from build123d import *

# Parameters (mm, degrees)
F0_R        = 3.81
F1_DEPTH    = 3.175
F2_R        = 10.16
F3_R        = 6.35
F4_T1_DEPTH = 25.1335533113
F5_R        = 6.35


# Not quite as in the source:
# - a fillet or chamfer that OpenCascade refuses, or shapes differently, is made with other operations: its cross-section is extruded or revolved along the edge and cut away or added


with BuildPart() as f1:
    # F0 (on Front) → F1 (new body, symmetric)
    with BuildSketch(Plane.XZ):
        Polygon((-49.1121449284, -23.3316957779), (-52.2871449284, -23.3316957779), (-52.2871449284, -97.4421674833), (1.6878550716, -97.4421674833), (1.6878550716, -23.3316957779), (-1.4871449284, -23.3316957779), (-1.4871449284, 87.3682325167), (-14.1871449284, 87.3682325167), (-14.1871449284, 156.5578325167), (-22.1246449284, 156.5578325167), (-22.1246449284, 29.5578325167), (-28.4746449284, 29.5578325167), (-28.4746449284, 156.5578325167), (-36.4121449284, 156.5578325167), (-36.4121449284, 87.3682325167), (-49.1121449284, 87.3682325167), align=None)
        with Locations((-38.7933949284, -84.7421674833)):
            Circle(F0_R, mode=Mode.SUBTRACT)
        with Locations((-11.8185949284, -84.7421674833)):
            Circle(F0_R, mode=Mode.SUBTRACT)
    extrude(amount=F1_DEPTH, both=True)

    # F2
    f2_edges = [f1.edges().sort_by_distance(p)[0] for p in [
        (-1.487145, 0, 87.368233),
        (-49.112145, 0, 87.368233),
    ]]
    fillet(f2_edges, radius=F2_R)

    # F3
    f3_edges = [f1.edges().sort_by_distance(p)[0] for p in [
        (-14.187145, 0, 156.557833),
        (-36.412145, 0, 156.557833),
    ]]
    fillet(f3_edges, radius=F3_R)

    # F4: fillet of radius 3.81 on 2 edges, made by hand

    # F4_s2 → F4_t1 (cut)
    with BuildSketch(Plane.XZ.offset(-12.5667766557)):
        with BuildLine():
            ThreePointArc((-49.1121449284, -23.3316957779), (-51.3870804947, -24.6290620154), (-52.2871449284, -27.0884064402))
            Line((-52.2871449284, -27.0884064402), (-52.2871449284, -23.3316957779))
            Line((-52.2871449284, -23.3316957779), (-49.1121449284, -23.3316957779))
        make_face()
        with BuildLine():
            ThreePointArc((1.6878550716, -27.0884064402), (0.7877906379, -24.6290620154), (-1.4871449284, -23.3316957779))
            Line((-1.4871449284, -23.3316957779), (1.6878550716, -23.3316957779))
            Line((1.6878550716, -23.3316957779), (1.6878550716, -27.0884064402))
        make_face()
    extrude(amount=F4_T1_DEPTH, mode=Mode.SUBTRACT)

    # F5
    f5_edges = [f1.edges().sort_by_distance(p)[0] for p in [
        (-52.287145, 0, -97.442167),
        (1.687855, 0, -97.442167),
    ]]
    fillet(f5_edges, radius=F5_R)


solid = f1.part
Part model, mm, in its own coordinate system. A direction names the side the tool comes from. Round coordinates to 2 decimals unless told otherwise and drop trailing zeros. Loops run counter-clockwise (first coordinate to the right, second up) from the corner with the lowest first, then second, coordinate; pieces in that order, holes last. Notation, with made-up numbers: (46.5, -10) - (52.5, -10) arc R38 cw to (52.5, 29) - close; hole circle Ø9 at (43, 22). An arc over 180 degrees is marked (long way). Answer as a JSON object with one key per item and string values.
Item 1: Pin check, flat tips, straight feed: pin 1 (1.9 mm diameter, centred on y = 0, z = 20.5, fed in from +X); pin 2 (3 mm diameter, centred on y = 0.5, z = 105, fed in from -X); pin 3 (2 mm diameter, centred on x = -38, y = -1.5, fed in from +Z). Stop position of each tip, or through.
Output:
{"pin 1": "x = -1.49", "pin 2": "x = -36.41", "pin 3": "z = 87.37"}
Item 2: Tool access for faces 1 (the face through (-36.412, 0, 119)), 2 (the face through (-0.12, -0.04, -95.53)), 3 (the face through (-14.187, 0, 118)), 4 (the face through (-25, 0, 29.558)): list every direction of +Z, -Z, +X, -X, +Y, -Y with a clear straight run to the whole face (end or side of a thin tool).
Output:
{"face 1": "+Z, -X, +Y, -Y", "face 2": "-Z, +X, +Y, -Y", "face 3": "+Z, +X, +Y, -Y", "face 4": "+Z, +Y, -Y"}
Item 3: Band-saw the part on A-A on y = 1.75. List the corners of the cut face in (x, z), plus the area to 3 significant figures.
Output:
{"outline": "(-52.29, -91.09) arc R6.35 ccw to (-45.94, -97.44) - (-4.66, -97.44) arc R6.35 ccw to (1.69, -91.09) - (1.69, -27.09) arc R3.81 ccw to (-1.49, -23.33) - (-1.49, 77.21) arc R10.16 ccw to (-11.65, 87.37) - (-14.19, 87.37) - (-14.19, 150.21) arc R6.35 ccw to (-20.54, 156.56) - (-22.12, 156.56) - (-22.12, 29.56) - (-28.47, 29.56) - (-28.47, 156.56) - (-30.06, 156.56) arc R6.35 ccw to (-36.41, 150.21) - (-36.41, 87.37) - (-38.95, 87.37) arc R10.16 ccw to (-49.11, 77.21) - (-49.11, -23.33) arc R3.81 ccw to (-52.29, -27.09) - close; hole circle Ø7.62 at (-38.79, -84.74); hole circle Ø7.62 at (-11.82, -84.74)", "area": "9,830 mm2"}
Item 4: Band-saw the part on B-B on z = 10. List the corners of the cut face in (x, y) (3 decimals).
Output:
{"outline": "(-49.112, -3.175) - (-1.487, -3.175) - (-1.487, 3.175) - (-49.112, 3.175) - close"}
Item 5: Wall check: L1, parallel to X at y = 0.75, z = -87; L2, parallel to X at y = 2.5, z = 137.5; L3, parallel to Z at x = -11.5, y = 0.5. Give the ranges that are in metal, low to high.
Output:
{"L1": "-52.29 to -41.86, -35.72 to -14.89, -8.75 to 1.69", "L2": "-36.41 to -28.47, -22.12 to -14.19", "L3": "-97.44 to -88.54, -80.95 to 87.37"}
